Build history of the part. All positions in model axes, mm. Face numbers are marked on the shaded views. A direction names the side the tool comes from. Round coordinates to 2 decimals unless told otherwise and drop trailing zeros. Write each loop counter-clockwise with the first axis right and the second up, starting at its lowest first coordinate (ties: lowest second). Pieces come first, ordered by that corner, then holes. Notation, with made-up numbers: (71, 71) - (106, 71) arc R12 cw to (106, 84) - close; hole circle Ø1 at (89.5, 22). An arc over 180 degrees is marked (long way). Write each question's results on one line, items separated by ' | '.
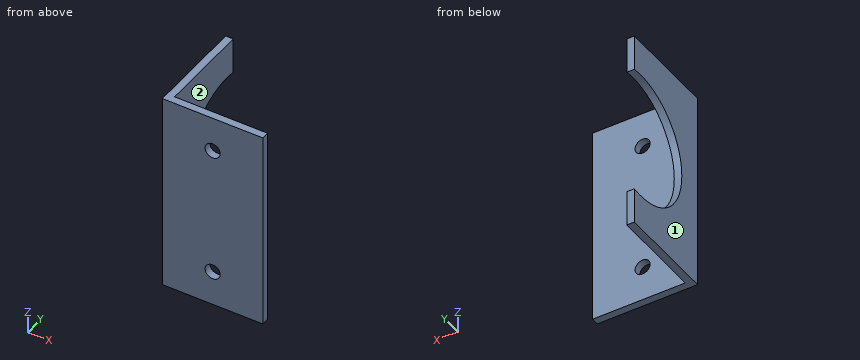
from build123d import *

# Parameters (mm, degrees)
EXTRUSION1_DEPTH = 40
ESQUISSE2_R      = 13
EXTRUSION2_DEPTH = 30
ESQUISSE3_R      = 1.5
EXTRUSION3_DEPTH = 49.396797415


with BuildPart() as part:
    # Esquisse1 → Extrusion1 (new body)
    with BuildSketch(Plane.XY):
        Polygon((0, 0), (0, 20), (1.5, 20), (1.5, 1.5), (20, 1.5), (20, 0), align=None)
    extrude(amount=EXTRUSION1_DEPTH)

    # Esquisse2 → Extrusion2 (cut)
    with BuildSketch(Plane(origin=(1.5, 0, 0), x_dir=(0, 0, -1), z_dir=(1, 0, 0))):
        with Locations((-20, 18)):
            Circle(ESQUISSE2_R)
    extrude(amount=-EXTRUSION2_DEPTH, mode=Mode.SUBTRACT)

    # Esquisse3 → Extrusion3 (cut, through all)
    with BuildSketch(Plane(origin=(0, 1.5, 0), x_dir=(-1, 0, 0), z_dir=(0, 1, 0))):
        with Locations((-10, 33)):
            Circle(ESQUISSE3_R)
        with Locations((-10, 7)):
            Circle(ESQUISSE3_R)
    extrude(amount=-EXTRUSION3_DEPTH, mode=Mode.SUBTRACT)


solid = part.part
(1) Tool access for the marked faces 1 and 2: list every direction of +Z, -Z, +X, -X, +Y, -Y with a clear straight run to the whole face (end or side of a thin tool).
Worked answers:
face 1: +Z, -Z, -X, +Y, -Y | face 2: +Z, -Z, +X, +Y
(2) Slice it at C-C, the plane z = 20. Write the cut outline in (x, y).
Worked answers:
outline: (0, 0) - (20, 0) - (20, 1.5) - (1.5, 1.5) - (1.5, 5) - (0, 5) - close
(3) Slice it at A-A, the plane x = 10. Write the cut outline in (y, z), and give its area (3 significant figures).
Worked answers:
outline: (0, 0) - (1.5, 0) - (1.5, 5.5) - (0, 5.5) - close; (0, 8.5) - (1.5, 8.5) - (1.5, 31.5) - (0, 31.5) - close; (0, 34.5) - (1.5, 34.5) - (1.5, 40) - (0, 40) - close | area: 51.0 mm2
(4) Slice it at D-D, the plane y = 16.75. Write the cut outline in (x, z), and give its area (3 significant figures).
Worked answers:
outline: (0, 0) - (1.5, 0) - (1.5, 7.06) - (0, 7.06) - close; (0, 32.94) - (1.5, 32.94) - (1.5, 40) - (0, 40) - close | area: 21.2 mm2
(5) Flat gauge pins, fed straight in: pin 1 Ø3 at (y, z) = (17, 29.5) entering from -X; pin 2 Ø5 at (x, z) = (10, 25.5) entering from +Y; pin 3 Ø9.5 at (y, z) = (8, 17) entering from +X. Where does each tip first touch, or does it go through?
Worked answers:
pin 1: passes through | pin 2: stops at y = 1.5 | pin 3: stops at x = 1.5
(6) Drill centre lines: probe 1 along Z at (x, y) = (10, 0.7); probe 2 along Z at (x, y) = (0.6, 18); probe 3 along X at (y, z) = (6.5, 26.5). Where is each one in solid material? Low to high. Write a range as [from, to].
Worked answers:
probe 1: z = [0, 5.5], [8.5, 31.5], [34.5, 40] | probe 2: z = [0, 7], [33, 40] | probe 3: x = [0, 1.5]
(7) Slice it at B-B, the plane y = 11.25. Write the cut outline in (x, z).
Worked answers:
outline: (0, 0) - (1.5, 0) - (1.5, 8.89) - (0, 8.89) - close; (0, 31.11) - (1.5, 31.11) - (1.5, 40) - (0, 40) - close
